```python
from build123d import *

# Parameters (mm, degrees)
SKETCH2_R               = 90
SKETCH2_R_2             = 38
BOSS_EXTRUDE1_DEPTH     = 100
SKETCH2_2_R             = 38
CUT_EXTRUDE1_DEPTH      = 101.0000001
CUT_EXTRUDE1_DEPTH_BACK = 101.0000001


with BuildPart() as part:
    # Sketch1 → Revolve2 (revolve)
    with BuildSketch(Plane.XY):
        Polygon((1825, 0), (1825, 75), (200, 75), (200, 90), (0, 90), (0, 51), (1750, 51), (1750, 0), align=None)
    revolve(axis=Axis((0, 0, 0), (1, 0, 0)))

    # Sketch2 → Boss-Extrude1 (add, symmetric)
    with BuildSketch(Plane.XY):
        with Locations((1825, 0)):
            Circle(SKETCH2_R)
        with Locations((1825, 0)):
            Circle(SKETCH2_R_2, mode=Mode.SUBTRACT)
    extrude(amount=BOSS_EXTRUDE1_DEPTH, both=True)

    # Sketch2_2 → Cut-Extrude1 (cut, two sides)
    with BuildSketch(Plane.XY) as cut_extrude1_sk:
        with Locations((1825, 0)):
            Circle(SKETCH2_2_R)
    extrude(amount=CUT_EXTRUDE1_DEPTH, mode=Mode.SUBTRACT)
    extrude(cut_extrude1_sk.sketch, amount=-CUT_EXTRUDE1_DEPTH_BACK, mode=Mode.SUBTRACT)


solid = part.part
```
Design review of the part built by this model. Coordinates are the model's own, in mm. A direction names the side the tool comes from. Give positions to 0.01 mm unless a question says otherwise; leave off trailing zeros. Loops run counter-clockwise (first coordinate to the right, second up) from the corner with the lowest first, then second, coordinate; pieces in that order, holes last. Notation, with made-up numbers: (26, -29) -> (52, -29) arc R31 ccw to (52, -5) -> close; hole circle Ø4 at (-26, 64.25). An arc over 180 degrees is marked (long way). Write each question's results on one line, items separated by ' | '.
Q1. The part is to be moulded in two halves that separate along X. For faces 4 (the face through (976.599, -9.764, 74.362)), 5 (the face through (98.6, 41.53, -79.845)), 6 (the face through (1860.102, -14.554, -1.4)), 7 (the face through (0, 39, -39)), say which applies: +X half, -X half, draft (parallel to the pull), parting line (faces both ways), or undercut.
Reply:
face 4: undercut | face 5: draft | face 6: undercut | face 7: -X half
Q2. Take a section at B-B, the plane y = 0. Write out the cut boundary in (x, z), plus the area to 3 significant figures.
Reply:
outline: (0, -90) -> (200, -90) -> (200, -75) -> (1735, -75) -> (1735, -100) -> (1787, -100) -> (1787, 100) -> (1735, 100) -> (1735, 75) -> (200, 75) -> (200, 90) -> (0, 90) -> (0, 51) -> (1735, 51) -> (1735, -51) -> (0, -51) -> close; (1863, -100) -> (1915, -100) -> (1915, 100) -> (1863, 100) -> close | area: 110,000 mm²
Q3. Take a section at C-C, the plane z = -32.5. Write out the cut boundary in (x, y), plus the area to 3 significant figures.
Reply:
outline: (0, -83.93) -> (200, -83.93) -> (200, -67.59) -> (1765.58, -67.59) arc R90 ccw (long way) to (1765.58, 67.59) -> (200, 67.59) -> (200, 83.93) -> (0, 83.93) -> (0, 39.3) -> (1744.04, 39.3) arc R90 ccw to (1744.04, -39.3) -> (0, -39.3) -> close; hole circle Ø76 at (1825, 0) | area: 127,000 mm²
Q4. Take a section at A-A, the plane x = 1825. Write out the cut boundary in (y, z).
Reply:
outline: (-90, -100) -> (-38, -100) -> (-38, 100) -> (-90, 100) -> close; (38, -100) -> (90, -100) -> (90, 100) -> (38, 100) -> close
Q5. For pin 1 Ø5 at (x, z) = (1110, 59) entering from -Y; pin 2 Ø3 at (y, z) = (66, -66.5) entering from -X; pin 3 Ø3 at (x, z) = (1255.5, -51) entering from -Y, all flat-tipped, find the tip position at first contact; note any pin that passes through.
Reply:
pin 1: stops at y = -49.32 | pin 2: stops at x = 1762.23 | pin 3: stops at y = -56.34
Q6. Take a section at D-D, the plane x = 566.5. Write out the cut boundary in (y, z), plus the area to 3 significant figures.
Reply:
outline: circle Ø150 at (0, 0); hole circle Ø102 at (0, 0) | area: 9,500 mm²
Q7. Wall thickness on L1, parallel to Y at x = 1825, z = -28.5; L2, parallel to Z at x = 676, y = 0; L3, parallel to Y at x = 860, z = 27.5: over which ranges is each line inside the solid? List them lowest first.
Reply:
L1: y = -90 to -38, 38 to 90 | L2: z = -75 to -51, 51 to 75 | L3: y = -69.78 to -42.95, 42.95 to 69.78
Q8. Machinability: for faces 1 (the face through (1864, 1, 100)), 2 (the face through (887.25, -11.056, -49.787)), 3 (the face through (200, 20, 74)), which of the approach directions +Z, -Z, +X, -X, +Y, -Y give a long, thin tool a straight path to every point of the face, cutting with its end or side? Answer none if there is none.
Reply:
face 1: +Z, +X, -X, +Y, -Y | face 2: -X | face 3: none
